The listing builds one solid part. Answer for the finished solid, in the listing's coordinates (mm). A direction names the side the tool comes from. Coordinates: 2 decimals unless noted, no trailing zeros. Write each loop counter-clockwise with the first axis right and the second up, starting at its lowest first coordinate (ties: lowest second). Pieces come first, ordered by that corner, then holes.
(1) Given P1, Ø4.5, axis at x = 6, z = 65, coming from the -Y side; P2, Ø5.5, axis at x = 6, z = -65, coming from the +Y side; P3, Ø4, axis at x = 2.5, y = 50, coming from the +Z side, each flat-ended and moving along its own axis, determine where each tip first touches the part or whether it passes through.
(2) The part is cut by section C-C on y = -53. Determine the outline of the cut face in (x, z), plus the area to 3 significant figures.
(3) Which of the six approach directions +Z, -Z, +X, -X, +Y, -Y give full straight-line access (tool end or side, diameter ignored) to faces 5 (the flat face through (6, -18, -72.5)), 6 (the cylindrical face through (4.929, -54.759, -68.402))?
(4) Straight lines are drawn through the part: line 1 (Y direction, x = 8, z = 26); line 2 (Z direction, x = 6, y = -60.5); line 3 (Y direction, x = 5.25, z = 1.5). For each, find the intervals that lie inside material, in ascending order.
(5) For a pull along X with two mould halves and no side action, classify faces 1 (the flat face through (0, -59, 1)), 2 (the cylindrical face through (5.92, 50.56, -49.9)), 3 (the flat face through (12, -59, 1)), 4 (the cylindrical face through (7.366, -54.759, 61.705)) as +X half, -X half, draft (parallel to the pull), parting line (faces both ways), or undercut.
(6) The part is cut by section D-D on x = 4.25. Give the number of separate pieces and of enclosed holes in the cut face, plus the area to 3 significant figures.
(7) The part is cut by section A-A on y = 0. Determine the outline of the cut face in (x, z), plus the area to 3 significant figures.
(8) The part is cut by section B-B on z = 0. Determine the outline of the cut face in (x, y), plus the area to 3 significant figures.
Autodesk Inventor part; units mm, degrees
ref_plane "YZ Plane" through (0, 0, 0) normal (1, 0, 0) x (0, 1, 0)
ref_plane "XZ Plane" through (0, 0, 0) normal (0, 1, 0) x (-1, 0, 0)
ref_plane "XY Plane" through (0, 0, 0) normal (0, 0, 1) x (1, 0, 0)
sketch "Sketch1" plane through (0, 0, 0) normal (1, 0, 0) x (0, 1, 0)
  line L0 (-65, -72.5) -> (65, -72.5)
  line L1 (65, -72.5) -> (65, 72.5)
  line L2 (65, 72.5) -> (-65, 72.5)
  line L3 (-65, 72.5) -> (-65, -72.5)
  line L4 (-65, -72.5) -> (65, 72.5) construction
  line L5 (65, -72.5) -> (-65, 72.5) construction
  point P0 (0, 0)
  dimension "d0" = 130
  dimension "d1" = 145
extrude "Extrusion1" add sketch "Sketch1" along normal blind 12
fillet "Fillet1" radius 35 2 edges at (6, 65, 72.5) (6, 65, -72.5)
sketch "Sketch2" plane through (0, -65, -72.5) normal (0, -1, 0) x (1, 0, 0)
  line L0 (0, 145) -> (12, 145)
  line L1 (0, 0) -> (12, 0)
  line L2 (12, 145) -> (12, 0)
  point P0 (0, 72.5)
  point P1 (6, 137.5)
  point P2 (6, 7.5)
  point P3 (6, 145)
  point P4 (6, 0)
  dimension "d5" = 7.5
  dimension "d6" = 7.5
  dimension "d7" = 6
  dimension "d8" = 6
hole "Hole1" at (6, -65, 65) at (6, -65, -65) direction (0, 1, 0) diameter 7.134 depth 20.2 tip angle 118
sketch "Sketch3" plane through (12, 0, 0) normal (1, 0, 0) x (0, 0, -1)
  circle A0 centre (0, 0) radius 57.5
  dimension "d16" = 115
extrude "Extrusion2" cut sketch "Sketch3" against normal blind 12
sketch "Sketch4" plane through (12, 0, 0) normal (1, 0, 0) x (0, 0, -1)
  circle A0 centre (0, 0) radius 67.5 construction
  line L0 (0, 0) -> (-82.2434, 82.2434) construction
  line L1 (0, 0) -> (116.3098, 0) construction
  point P0 (-47.7297, 47.7297)
  dimension "d19" = 135
  dimension "d20" = 135
hole "Hole2" at (12, 47.7297, 47.7297) direction (-1, 0, 0) diameter 7.134 depth 20.2 tip angle 118
pattern_circular "Circular Pattern1" count 4 over 360 about axis through (-10, 0, 0) along (1, 0, 0) of "Hole2"
properties part number "Gear_support"
Model answer:
1. P1: stops at y = -44.01
1. P2: stops at y = 54.75
1. P3: stops at z = 67.52
2. outline: (0, -72.5) - (12, -72.5) - (12, -22.3) - (0, -22.3) - close; (0, 22.3) - (12, 22.3) - (12, 72.5) - (0, 72.5) - close; hole circle Ø7.13 at (6, -65); hole circle Ø7.13 at (6, 65)
2. area: 1,120 mm2
3. face 5: -Z, +X, -X, +Y, -Y
3. face 6: -Y
4. line 1: y = -65 to -51.29, 51.29 to 65
4. line 2: z = -72.5 to -68.57, -61.43 to 61.43, 68.57 to 72.5
4. line 3: y = -65 to -57.48, 57.48 to 65
5. face 1: -X half
5. face 2: draft
5. face 3: +X half
5. face 4: undercut
6. separate pieces: 1
6. enclosed holes: 5
6. area: 7,520 mm2
7. outline: (0, -72.5) - (12, -72.5) - (12, -57.5) - (0, -57.5) - close; (0, 57.5) - (12, 57.5) - (12, 72.5) - (0, 72.5) - close
7. area: 360 mm2
8. outline: (0, -65) - (12, -65) - (12, -57.5) - (0, -57.5) - close; (0, 57.5) - (12, 57.5) - (12, 65) - (0, 65) - close
8. area: 180 mm2
